Read the model definition and answer for the solid it produces. Units are mm, in the model's axes. A direction names the side the tool comes from. Round coordinates to 2 decimals unless told otherwise and drop trailing zeros. Loops run counter-clockwise (first coordinate to the right, second up) from the corner with the lowest first, then second, coordinate; pieces in that order, holes last. Notation, with made-up numbers: M -23,31 L 4,31 A31 ccw 4,67 Z; hole C 24,-1 d11. An arc over 180 degrees is marked long. Write each question's results on one line, items separated by ' | '.
```python
from build123d import *

# Parameters (mm, degrees)
SKETCH1_R               = 101
SKETCH1_R_2             = 80
BOSS_EXTRUDE1_DEPTH     = 38
SKETCH3_R               = 27.5
CUT_EXTRUDE1_DEPTH      = 102
CUT_EXTRUDE1_DEPTH_BACK = 102
SKETCH4_R               = 5.25
CUT_EXTRUDE2_DEPTH      = 76
CIRPATTERN1_COUNT       = 8
CUT_EXTRUDE3_DEPTH      = 68
SKETCH6_R               = 101
SKETCH6_R_2             = 97.5
BOSS_EXTRUDE2_DEPTH     = 3
SKETCH7_R               = 97.5
CUT_EXTRUDE4_DEPTH      = 3


with BuildPart() as part:
    # Sketch1 → Boss-Extrude1 (new body, symmetric)
    with BuildSketch(Plane(origin=(0, 0, 0), x_dir=(1, 0, 0), z_dir=(0, 1, 0))):
        Circle(SKETCH1_R)
        Circle(SKETCH1_R_2, mode=Mode.SUBTRACT)
    extrude(amount=BOSS_EXTRUDE1_DEPTH, both=True)

    # Sketch3 → Cut-Extrude1 (cut, two sides)
    with BuildSketch(Plane.XY) as cut_extrude1_sk:
        with Locations((0, -5)):
            Circle(SKETCH3_R)
    extrude(amount=CUT_EXTRUDE1_DEPTH, mode=Mode.SUBTRACT)
    extrude(cut_extrude1_sk.sketch, amount=-CUT_EXTRUDE1_DEPTH_BACK, mode=Mode.SUBTRACT)

    # Sketch4 → Cut-Extrude2 (cut)
    with BuildSketch(Plane(origin=(0, 38, 0), x_dir=(1, 0, 0), z_dir=(0, 1, 0))):
        with Locations((-34.05882548, 82.225278394)):
            Circle(SKETCH4_R)
    cut_extrude2 = extrude(amount=-CUT_EXTRUDE2_DEPTH, mode=Mode.SUBTRACT)

    # CirPattern1: Cut-Extrude2 ×8 about axis
    cirpattern1_axis = Axis((0, 0, 0), (0, 1, 0))
    for i in range(1, CIRPATTERN1_COUNT):
        add(cut_extrude2.rotate(cirpattern1_axis, i * 360 / CIRPATTERN1_COUNT), mode=Mode.SUBTRACT)

    # Sketch5 → Cut-Extrude3 (cut)
    with BuildSketch(Plane.XZ.offset(38)):
        with BuildLine():
            Line((-72.5, 2), (72.5, 2))
            ThreePointArc((72.5, 2), (87.5, -13), (72.5, -28))
            Line((72.5, -28), (-72.5, -28))
            ThreePointArc((-72.5, -28), (-87.5, -13), (-72.5, 2))
        make_face()
    extrude(amount=-CUT_EXTRUDE3_DEPTH, mode=Mode.SUBTRACT)

    # Sketch6 → Boss-Extrude2 (add)
    with BuildSketch(Plane.XZ.offset(38)):
        Circle(SKETCH6_R)
        Circle(SKETCH6_R_2, mode=Mode.SUBTRACT)
    extrude(amount=BOSS_EXTRUDE2_DEPTH)

    # Sketch7 → Cut-Extrude4 (cut)
    with BuildSketch(Plane(origin=(0, 38, 0), x_dir=(1, 0, 0), z_dir=(0, 1, 0))):
        Circle(SKETCH7_R)
    extrude(amount=-CUT_EXTRUDE4_DEPTH, mode=Mode.SUBTRACT)


solid = part.part
```
1. Which of the six approach directions +Z, -Z, +X, -X, +Y, -Y give full straight-line access (tool end or side, diameter ignored) to faces 5 (the face through (39.185, -0.989, -83.36)), 6 (the face through (87.31, -4.48, -15.39)), 7 (the face through (-77.37, 36.52, 59.33))?
Completed:
face 5: +Y, -Y | face 6: -Y | face 7: +Y
2. Find section A-A, the plane x = 0. Give the vertices of the cut face in (y, z), then the cut area to 3 significant figures.
Completed:
outline: M -41,-101 L -32.5,-101 L -32.5,-80 L -38,-80 L -38,-97.5 L -41,-97.5 Z; M -41,97.5 L -38,97.5 L -38,80 L -32.5,80 L -32.5,101 L -41,101 Z; M 22.5,-101 L 38,-101 L 38,-97.5 L 35,-97.5 L 35,-80 L 22.5,-80 Z; M 22.5,80 L 35,80 L 35,97.5 L 38,97.5 L 38,101 L 22.5,101 Z | area: 798 mm2
3. Given P1, Ø5, axis at y = -7.5, z = -77, coming from the +X side; P2, Ø4, axis at y = -29, z = 78, coming from the -X side; P3, Ø3, axis at x = 59.5, y = 23, coming from the +Z side, each flat-ended and moving along its own axis, determine where each tip first touches the part or whether it passes through.
Completed:
P1: stops at x = 68.2 | P2: stops at x = -66.52 | P3: stops at z = 82.69
4. Find section B-B, the plane y = 1.5. Count the separate pieces of the cut face and the enclosed holes in it, then the cut area to 3 significant figures.
Completed:
separate pieces: 2 | enclosed holes: 8 | area: 8,610 mm2
5. Determine the mould class of faces 1 (the face through (-53, -41, 83)), 2 (the face through (46.61, -0.95, -89.6)), 3 (the face through (83.36, -0.989, 39.185)), 4 (the face through (7, 35, -80)) for opening direction Z: released by +Z, released by -Z, zero draft, split by the parting line, or undercut.
Completed:
face 1: zero draft | face 2: split by the parting line | face 3: undercut | face 4: undercut
6. Find the intervals of material crossed by L1, parallel to X at y = 36, z = 0; L2, parallel to Z at x = -86, y = 22; L3, parallel to X at y = 16, z = 0, in increasing order.
Completed:
L1: x = -101 to -97.5, 97.5 to 101 | L2: z = -52.96 to -37.71, -30.41 to -19.54, -6.46 to 30.41, 37.71 to 52.96 | L3: x = -101 to -80, 80 to 101
7. Find section C-C, the plane z = -51. Give the vertices of the cut face in (x, y).
Completed:
outline: M -87.18,-41 L -83.1,-41 L -83.1,-38 L -61.64,-38 L -61.64,35 L -83.1,35 L -83.1,38 L -87.18,38 Z; M 61.64,-38 L 83.1,-38 L 83.1,-41 L 87.18,-41 L 87.18,38 L 83.1,38 L 83.1,35 L 61.64,35 Z
